Autodesk Inventor part; units mm, degrees
ref_plane "YZ Plane" through (0, 0, 0) normal (1, 0, 0) x (0, 1, 0)
ref_plane "XZ Plane" through (0, 0, 0) normal (0, 1, 0) x (-1, 0, 0)
ref_plane "XY Plane" through (0, 0, 0) normal (0, 0, 1) x (1, 0, 0)
sketch "Esquisse1" plane through (0, 0, 0) normal (0, 1, 0) x (-1, 0, 0)
  line L0 (35, -30.5) -> (-35, -30.5)
  line L1 (-35, -30.5) -> (-35, 30.5)
  line L2 (-35, 30.5) -> (35, 30.5)
  line L3 (35, 30.5) -> (35, -30.5)
  point P0 (0, 0)
  dimension "d0" = 70
  dimension "d1" = 35
  dimension "d2" = 61
  dimension "d3" = 30.5
extrude "Extrusion1" add sketch "Esquisse1" along normal blind 1.6
sketch "Esquisse2" plane through (0, 1.6, 0) normal (0, 1, 0) x (1, 0, 0)
  line L0 (35, 30.5) -> (-35, 30.5)
  line L1 (-35, 30.5) -> (-23, 30.5)
  line L2 (-23, 30.5) -> (-23, 19.5)
  line L3 (-23, 19.5) -> (-35, 19.5)
  line L4 (-35, 19.5) -> (-35, 30.5)
  line L5 (35, 30.5) -> (23, 30.5)
  line L6 (23, 30.5) -> (23, 19.5)
  line L7 (23, 19.5) -> (35, 19.5)
  line L8 (35, 19.5) -> (35, 30.5)
  line L9 (-35, -30.5) -> (35, -30.5)
  line L10 (-20.5, -30.5) -> (23, -30.5)
  line L11 (-21.75, -30.5) -> (21.75, -30.5)
  line L12 (21.75, -30.5) -> (21.75, -18.5)
  line L13 (21.75, -18.5) -> (-21.75, -18.5)
  line L14 (-21.75, -18.5) -> (-21.75, -30.5)
  point P0 (0, 0)
  dimension "d6" = 12
  dimension "d7" = 12
  dimension "d8" = 11
  dimension "d11" = 43.5
  dimension "d12" = 21.75
  dimension "d13" = 12
extrude "Extrusion2" cut sketch "Esquisse2" against normal through all
fillet "Congé1" radius 1.5 12 edges at (-35, 0.8, 30.5) (-21.75, 0.8, 30.5) (-21.75, 0.8, 18.5) (21.75, 0.8, 18.5) (21.75, 0.8, 30.5) (35, 0.8, 30.5) (23, 0.8, -19.5) (23, 0.8, -30.5) (35, 0.8, -19.5) (-23, 0.8, -30.5) (-23, 0.8, -19.5) (-35, 0.8, -19.5)
sketch "Esquisse3" plane through (0, 1.6, 0) normal (0, 1, 0) x (1, 0, 0)
  line L0 (-25, 19) -> (-22.5, 19)
  line L1 (-22.5, 19) -> (-22.5, -29)
  line L2 (-22.5, -29) -> (-25, -29)
  line L3 (-25, -29) -> (-25, 19)
  line L4 (22.5, 19) -> (25, 19)
  line L5 (25, 19) -> (25, -20)
  line L6 (25, -20) -> (22.5, -20)
  line L7 (22.5, -20) -> (22.5, 19)
  line L8 (-35, 18) -> (-35, -29)
  line L9 (35, -29) -> (35, 18)
  line L10 (-24.5, 19.5) -> (-33.5, 19.5)
  line L11 (33.5, 19.5) -> (24.5, 19.5)
  point P0 (0, 0)
  dimension "d17" = 2.5
  dimension "d18" = 2.5
  dimension "d19" = 48
  dimension "d20" = 39
  dimension "d21" = 10
  dimension "d22" = 10
  dimension "d23" = 0.5
  dimension "d24" = 0.5
extrude "Extrusion3" add sketch "Esquisse3" along normal blind 10
sketch "Esquisse4" plane through (0, 0, 0) normal (0, -1, 0) x (1, 0, 0)
  line L0 (22.5, -19) -> (25, -19)
  line L1 (22.5, 20) -> (22.5, -19)
  line L2 (25, -19) -> (25, 20)
  line L3 (25, 20) -> (22.5, 20)
  line L4 (-25, 29) -> (-25, -19)
  line L5 (-25, -19) -> (-22.5, -19)
  line L6 (-22.5, -19) -> (-22.5, 29)
  line L7 (-22.5, 29) -> (-25, 29)
  point P0 (0, 0)
extrude "Extrusion4" add sketch "Esquisse4" along normal blind 2
equation "\"d7\" = d6"
equation "\"d18\" = d17"
equation "\"d22\" = d21"
equation "\"d24\" = d23"
properties part number "X-Nucleo-IKS01A1" material "Nylon, disulfure de molybdène"
The listing builds one solid part. Answer for the finished solid, in the listing's coordinates (mm). A direction names the side the tool comes from. Coordinates: 2 decimals unless noted, no trailing zeros. Write each loop counter-clockwise with the first axis right and the second up, starting at its lowest first coordinate (ties: lowest second). Pieces come first, ordered by that corner, then holes. Notation, with made-up numbers: (63, -33) -> (70, -33) arc R25 cw to (70, 0) -> close; hole circle Ø2 at (-23, -23). An arc over 180 degrees is marked (long way). One line per question, with ' | ' between items.
1. Section B-B (z = 6) is taken. Determine the outline of the cut face in (x, y), and give its area (3 significant figures).
Verdict:
outline: (-35, 0) -> (-25, 0) -> (-25, -2) -> (-22.5, -2) -> (-22.5, 0) -> (22.5, 0) -> (22.5, -2) -> (25, -2) -> (25, 0) -> (35, 0) -> (35, 1.6) -> (25, 1.6) -> (25, 11.6) -> (22.5, 11.6) -> (22.5, 1.6) -> (-22.5, 1.6) -> (-22.5, 11.6) -> (-25, 11.6) -> (-25, 1.6) -> (-35, 1.6) -> close | area: 172 mm^2
2. Section A-A (y = 10.75) is taken. Determine the outline of the cut face in (x, z).
Verdict:
outline: (-25, -19) -> (-22.5, -19) -> (-22.5, 29) -> (-25, 29) -> close; (22.5, -19) -> (25, -19) -> (25, 20) -> (22.5, 20) -> close
3. Straight lines are drawn through the part: line 1 (X direction, y = -0.75, z = 2.5); line 2 (Y direction, x = 4.5, z = -6.5); line 3 (X direction, y = 5.25, z = 21). For each, find the intervals that lie inside material, in ascending order.
Verdict:
line 1: x = -25 to -22.5, 22.5 to 25 | line 2: y = 0 to 1.6 | line 3: x = -25 to -22.5
4. Section D-D (z = -22) is taken. Determine the outline of the cut face in (x, y), and give its area (3 significant figures).
Verdict:
outline: (-23, 0) -> (23, 0) -> (23, 1.6) -> (-23, 1.6) -> close | area: 73.6 mm^2
5. Given pin 1 Ø2 at (x, z) = (-27.5, -4.5) entering from -Y; pin 2 Ø3 at (x, y) = (-10.5, 4.5) entering from -Z; pin 3 Ø5 at (y, z) = (4.5, 0) entering from +X; pin 4 Ø6 at (x, y) = (-23.5, 7) entering from +Z, each flat-ended and moving along its own axis, determine where each tip first touches the part or whether it passes through.
Verdict:
pin 1: stops at y = 0 | pin 2: passes through | pin 3: stops at x = 25 | pin 4: stops at z = 29
6. Which of the six approach directions +Z, -Z, +X, -X, +Y, -Y give full straight-line access (tool end or side, diameter ignored) to faces 1 (the flat face through (29, 1, -19.5)), 2 (the flat face through (24, 7, 20)), 3 (the flat face through (25, 7, 0)), 4 (the flat face through (-22.5, -1, 5))?
Verdict:
face 1: -Z, +X, +Y, -Y | face 2: +Z, +X, +Y | face 3: +Z, -Z, +X, +Y | face 4: +Z, -Z, -Y
7. Section C-C (x = -19) is taken. Determine the outline of the cut face in (y, z).
Verdict:
outline: (0, -30.5) -> (1.6, -30.5) -> (1.6, 18.5) -> (0, 18.5) -> close
